Autodesk Inventor part; units mm, degrees
ref_plane "YZ Plane" through (0, 0, 0) normal (1, 0, 0) x (0, 1, 0)
ref_plane "XZ Plane" through (0, 0, 0) normal (0, 1, 0) x (-1, 0, 0)
ref_plane "XY Plane" through (0, 0, 0) normal (0, 0, 1) x (1, 0, 0)
sketch "Sketch1" plane through (0, 0, 0) normal (0, 1, 0) x (-1, 0, 0)
  line L0 (478.912, 694) -> (-478.912, 694)
  line L1 (-478.912, 694) -> (-478.912, -694)
  line L2 (-478.912, -694) -> (478.912, -694)
  line L3 (478.912, -694) -> (478.912, 694)
  line L4 (478.912, 694) -> (-478.912, -694) construction
  line L5 (-478.912, 694) -> (478.912, -694) construction
  line L6 (458.912, 674) -> (-458.912, 674)
  line L7 (-458.912, 674) -> (-458.912, -674)
  line L8 (-458.912, -674) -> (458.912, -674)
  line L9 (458.912, -674) -> (458.912, 674)
  line L10 (458.912, 674) -> (-458.912, -674) construction
  line L11 (-458.912, 674) -> (458.912, -674) construction
  line L12 (438.912, 400) -> (458.912, 400)
  line L13 (458.912, 400) -> (458.912, -400)
  line L14 (458.912, -400) -> (438.912, -400)
  line L15 (438.912, -400) -> (438.912, 400)
  line L16 (438.912, 400) -> (458.912, -400) construction
  line L17 (458.912, 400) -> (438.912, -400) construction
  line L18 (-458.912, 400) -> (-438.912, 400)
  line L19 (-438.912, 400) -> (-438.912, -400)
  line L20 (-438.912, -400) -> (-458.912, -400)
  line L21 (-458.912, -400) -> (-458.912, 400)
  line L22 (-458.912, 400) -> (-438.912, -400) construction
  line L23 (-438.912, 400) -> (-458.912, -400) construction
  line L24 (-350, 674) -> (350, 674)
  line L25 (350, 674) -> (350, 654)
  line L26 (350, 654) -> (-350, 654)
  line L27 (-350, 654) -> (-350, 674)
  line L28 (-350, 674) -> (350, 654) construction
  line L29 (350, 674) -> (-350, 654) construction
  line L30 (350, -654) -> (-350, -654)
  line L31 (-350, -654) -> (-350, -674)
  line L32 (-350, -674) -> (350, -674)
  line L33 (350, -674) -> (350, -654)
  line L34 (350, -654) -> (-350, -674) construction
  line L35 (-350, -654) -> (350, -674) construction
  point P0 (0, 0)
  point P1 (448.912, 0)
  point P2 (458.912, 0)
  point P3 (-448.912, 0)
  point P4 (-458.912, 0)
  point P5 (0, 664)
  point P6 (0, -664)
  point P7 (0, 674)
  point P8 (0, -674)
  dimension "d0" = 957.824
  dimension "d1" = 1388
  dimension "d2" = 917.824
  dimension "d3" = 1348
  dimension "d4" = 20
  dimension "d5" = 800
  dimension "d6" = 20
  dimension "d7" = 800
  dimension "d8" = 700
  dimension "d9" = 20
  dimension "d10" = 700
  dimension "d11" = 20
extrude "Extrusion6" add sketch "Sketch1" along normal blind 50 contours L25 L26 L27 L6 | L9 L14 L15 L12 | L18 L19 L20 L7 | L8 L31 L30 L33
extrude "Extrusion7" add sketch "Sketch1" along normal blind 100
sketch "Sketch2" plane through (478.912, 0, 694) normal (1, 0, 0) x (0, 0, -1)
  line L0 (0, 0) -> (0, 100)
  line L1 (0, 100) -> (1388, 100)
  point P0 (694, 0)
  point P1 (40, 75)
  dimension "d40" = 40
  dimension "d41" = 25
hole "Hole1" at (478.912, 75, 654) direction (-1, 0, 0) diameter 8 end through all
sketch "Sketch3" plane through (478.912, 0, 694) normal (1, 0, 0) x (0, 0, -1)
  line L0 (0, 0) -> (0, 100)
  line L1 (0, 0) -> (1388, 0)
  point P0 (694, 0)
  point P1 (40, 25)
  dimension "d42" = 40
  dimension "d43" = 25
hole "Hole2" at (478.912, 25, 654) direction (-1, 0, 0) diameter 8 end through all
sketch "Sketch4" plane through (478.912, 0, 694) normal (1, 0, 0) x (0, 0, -1)
  line L0 (1388, 0) -> (1388, 100)
  line L1 (0, 100) -> (1388, 100)
  point P0 (694, 0)
  point P1 (1348, 75)
  dimension "d58" = 40
  dimension "d59" = 25
hole "Hole3" at (478.912, 75, -654) direction (-1, 0, 0) diameter 8 end through all
sketch "Sketch5" plane through (478.912, 0, 694) normal (1, 0, 0) x (0, 0, -1)
  line L0 (1388, 0) -> (1388, 100)
  line L1 (0, 0) -> (1388, 0)
  point P0 (694, 0)
  point P1 (1348, 25)
  dimension "d60" = 40
  dimension "d61" = 25
hole "Hole4" at (478.912, 25, -654) direction (-1, 0, 0) diameter 8 end through all
sketch "Sketch6" plane through (-478.912, 0, 694) normal (0, 0, 1) x (1, 0, 0)
  line L0 (0, 100) -> (957.824, 100)
  line L1 (957.824, 0) -> (957.824, 100)
  line L2 (0, 0) -> (957.824, 0)
  point P0 (478.912, 0)
  point P1 (917.824, 75)
  point P2 (917.824, 25)
  dimension "d69" = 25
  dimension "d70" = 40
  dimension "d71" = 40
  dimension "d72" = 25
hole "Hole5" at (438.912, 75, 694) at (438.912, 25, 694) direction (0, 0, -1) diameter 8 end through all
sketch "Sketch7" plane through (-478.912, 0, 694) normal (0, 0, 1) x (1, 0, 0)
  line L0 (0, 0) -> (0, 100)
  line L1 (0, 100) -> (957.824, 100)
  point P0 (478.912, 0)
  point P1 (40, 75)
  dimension "d87" = 40
  dimension "d88" = 25
hole "Hole6" at (-438.912, 75, 694) direction (0, 0, -1) diameter 8 end through all
sketch "Sketch8" plane through (-478.912, 0, 694) normal (0, 0, 1) x (1, 0, 0)
  line L0 (0, 0) -> (0, 100)
  line L1 (0, 0) -> (957.824, 0)
  point P0 (478.912, 0)
  point P1 (40, 25)
  dimension "d89" = 40
  dimension "d90" = 25
hole "Hole7" at (-438.912, 25, 694) direction (0, 0, -1) diameter 8 end through all
properties part number "tub floor 1"
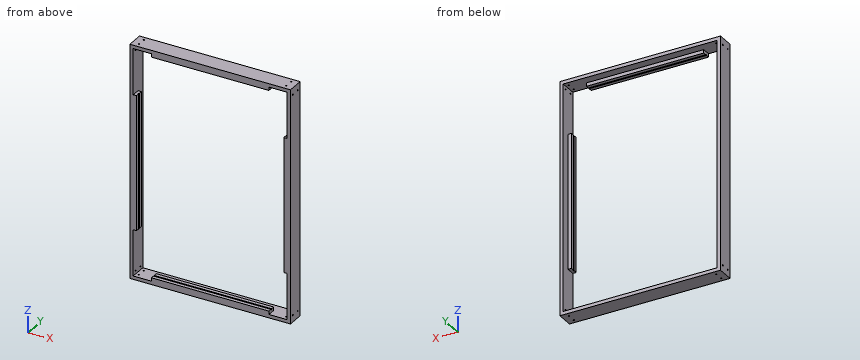
Work out the finished part from the listing and answer in its coordinate system (mm). Round coordinates to 2 decimals unless told otherwise and drop trailing zeros. Order: outer loops, then holes, each group sorted by start corner. A loop starts at its lowest first (then second) coordinate and runs counter-clockwise, first axis right, second up.
Q1. A cutting plane is placed at A-A, the plane x = -113. Determine the outline of the cut face in (y, z).
Solution:
outline: (0, -694) - (100, -694) - (100, -674) - (50, -674) - (50, -654) - (29, -654) arc R4 cw to (21, -654) - (0, -654) - close; (0, 654) - (21, 654) arc R4 cw to (29, 654) - (50, 654) - (50, 674) - (100, 674) - (100, 694) - (0, 694) - close
Q2. Given pin 1 Ø9 at (y, z) = (25, 654) entering from +X; pin 2 Ø5 at (y, z) = (25, -654) entering from +X, each flat-ended and moving along its own axis, determine where each tip first touches the part or whether it passes through.
Solution:
pin 1: stops at x = 478.91
pin 2: passes through
Q3. A cutting plane is placed at B-B, the plane z = 249. Determine the outline of the cut face in (x, y), then the cut area to 3 significant figures.
Solution:
outline: (-478.91, 0) - (-438.91, 0) - (-438.91, 21) arc R4 cw to (-438.91, 29) - (-438.91, 50) - (-458.91, 50) - (-458.91, 100) - (-478.91, 100) - close; (438.91, 0) - (478.91, 0) - (478.91, 100) - (458.91, 100) - (458.91, 50) - (438.91, 50) - (438.91, 29) arc R4 cw to (438.91, 21) - close
area: 5,950 mm2
Q4. Find the intervals of material crossed by line 1 along X through (y, z) = (25, 679.25); line 2 along Z through (x, y) = (-472, 25); line 3 along Z through (x, y) = (249.5, 52), in increasing order.
Solution:
line 1: x = -478.91 to -442.91, -434.91 to 434.91, 442.91 to 478.91
line 2: z = -694 to -658, -650 to 650, 658 to 694
line 3: z = -694 to -674, 674 to 694
